Part model, mm, in its own coordinate system. Face numbers are marked on the shaded views. A direction names the side the tool comes from. Coordinates: 2 decimals unless noted, no trailing zeros. Write each loop counter-clockwise with the first axis right and the second up, starting at its lowest first coordinate (ties: lowest second). Pieces come first, ordered by that corner, then holes. Notation, with made-up numbers: (-9.75, 87) -> (49.25, 87) arc R25 cw to (49.25, 104) -> close; hole circle Ø9 at (51.5, 2). An arc over 180 degrees is marked (long way). Write item = value, one per line.
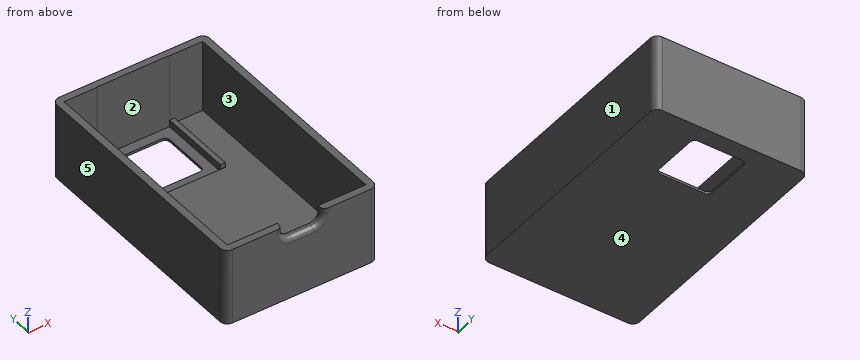
from build123d import *

# Parameters (mm, degrees)
F0_W      = 32
F0_H      = 51.5
F1_DEPTH  = 1
F2_DEPTH  = 16
F3_R      = 1.5
F4_W      = 8.5
F4_H      = 3
F5_DEPTH  = 5
F6_R      = 2
F7_R      = 1
F0_W_2    = 15.2
F0_H_2    = 13.6
F0_W_3    = 11.1999999404
F0_H_3    = 11.1999999404
F0_H_4    = 0.1
F0_H_5    = 1.5
F8_DEPTH  = 0.5
F9_R      = 1
F10_W     = 1
F10_H     = 15.1
F11_DEPTH = 1


with BuildPart() as f1:
    # F0 (on Top) → F1 (new body)
    with BuildSketch(Plane.XY):
        Rectangle(F0_W, F0_H)
        Polygon((7.6, 24.35), (7.6, 24.25), (14.5, 24.25), (14.5, -24.25), (-14.5, -24.25), (-14.5, 24.25), (-7.6, 24.25), (-7.6, 24.35), align=None, mode=Mode.SUBTRACT)
        Polygon((13, 22.75), (13, -22.75), (-13, -22.75), (-13, 22.75), (-7.6, 22.75), (-7.6, 24.25), (-14.5, 24.25), (-14.5, -24.25), (14.5, -24.25), (14.5, 24.25), (7.6, 24.25), (7.6, 22.75), align=None)
        Polygon((-13, -22.75), (13, -22.75), (13, 22.75), (7.6, 22.75), (7.6, 9.15), (-7.6, 9.15), (-7.6, 22.75), (-13, 22.75), align=None)
    extrude(amount=F1_DEPTH)

    # F0 (on Top) → F2 (join)
    with BuildSketch(Plane.XY):
        Rectangle(F0_W, F0_H)
        Polygon((7.6, 24.35), (7.6, 24.25), (14.5, 24.25), (14.5, -24.25), (-14.5, -24.25), (-14.5, 24.25), (-7.6, 24.25), (-7.6, 24.35), align=None, mode=Mode.SUBTRACT)
    extrude(amount=F2_DEPTH)

    # F3
    f3_edges = [f1.edges().sort_by_distance(p)[0] for p in [
        (-16, -25.75, 8),
        (16, -25.75, 8),
        (-16, 25.75, 8),
        (16, 25.75, 8),
    ]]
    fillet(f3_edges, radius=F3_R)

    # F4 (on face) → F5 (cut)
    with BuildSketch(Plane.XZ.offset(25.75)):
        with Locations((0.25, 14.5)):
            Rectangle(F4_W, F4_H)
    extrude(amount=-F5_DEPTH, mode=Mode.SUBTRACT)

    # F6
    f6_edges = [f1.edges().sort_by_distance(p)[0] for p in [
        (-4, -25, 13),
        (4.5, -25, 13),
    ]]
    fillet(f6_edges, radius=F6_R)

    # F7
    f7_edges = [f1.edges().sort_by_distance(p)[0] for p in [
        (-3.414214, -25.75, 13.585786),
        (0.25, -25.75, 13),
    ]]
    fillet(f7_edges, radius=F7_R)

    # F0 (on Top) → F8 (join)
    with BuildSketch(Plane.XY):
        with Locations((0, 15.95)):
            Rectangle(F0_W_2, F0_H_2)
        with Locations((0, 16.75)):
            Rectangle(F0_W_3, F0_H_3, mode=Mode.SUBTRACT)
        with Locations((0, 24.3)):
            Rectangle(F0_W_2, F0_H_4)
        with Locations((0, 23.5)):
            Rectangle(F0_W_2, F0_H_5)
    extrude(amount=F8_DEPTH)

    # F9
    f9_edges = [f1.edges().sort_by_distance(p)[0] for p in [
        (5.6, 11.15, 0.25),
        (-5.6, 11.15, 0.25),
        (5.6, 22.35, 0.25),
        (-5.6, 22.35, 0.25),
    ]]
    fillet(f9_edges, radius=F9_R)

    # F10 (on face) → F11 (join)
    with BuildSketch(Plane.XY.offset(1)):
        with Locations((-8.1, 16.7)):
            Rectangle(F10_W, F10_H)
        with Locations((8.1, 16.7)):
            Rectangle(F10_W, F10_H)
    extrude(amount=F11_DEPTH)


solid = f1.part
Q1. Saw through at A-A on z = 10. Give the cut face in (x, y), and give its area (3 significant figures).
Model answer:
outline = (-16, -24.25) arc R1.5 ccw to (-14.5, -25.75) -> (14.5, -25.75) arc R1.5 ccw to (16, -24.25) -> (16, 24.25) arc R1.5 ccw to (14.5, 25.75) -> (-14.5, 25.75) arc R1.5 ccw to (-16, 24.25) -> close; hole (-14.5, -24.25) -> (14.5, -24.25) -> (14.5, 24.25) -> (7.6, 24.25) -> (7.6, 24.35) -> (-7.6, 24.35) -> (-7.6, 24.25) -> (-14.5, 24.25) -> close
area = 238 mm²
Q2. Pin check, flat tip, straight feed: pin 1 (12 mm diameter, centred on x = -1.5, y = 10, fed in from +Z). Stop position of the tip, or through.
Model answer:
pin_1 = 1
Q3. Which spindle directions (+Z, -Z, +X, -X, +Y, -Y) get a long thin tool onto all of the face, cutting with end or side? Do the marked faces 1 and 2. Say none if no direction does.
Model answer:
face_1 = +Z, -Z, +X, +Y, -Y
face_2 = +Z
Q4. Saw through at B-B on y = -2. Give the cut face in (x, z).
Model answer:
outline = (-16, 0) -> (16, 0) -> (16, 16) -> (14.5, 16) -> (14.5, 1) -> (-14.5, 1) -> (-14.5, 16) -> (-16, 16) -> close
Q5. Saw through at C-C on x = 12.5. Give the cut face in (y, z), and give its area (3 significant figures).
Model answer:
outline = (-25.75, 0) -> (25.75, 0) -> (25.75, 16) -> (24.25, 16) -> (24.25, 1) -> (-24.25, 1) -> (-24.25, 16) -> (-25.75, 16) -> close
area = 96.5 mm²
Q6. Probe line 1 (X direction, y = -20, z = 9.5); line 2 (Y direction, x = -11.5, z = 4); line 3 (Y direction, x = 7.5, z = 9.75). List the from-to ranges inside material, lowest first. Write a range as from..to.
Model answer:
line_1 = -16..-14.5, 14.5..16
line_2 = -25.75..-24.25, 24.25..25.75
line_3 = -25.75..-24.25, 24.35..25.75
Q7. Mould opens along X. For the marked faces 3, 4 and 5 say: released by +X, released by -X, zero draft, split by the parting line, or undercut.
Model answer:
face_3 = undercut
face_4 = zero draft
face_5 = released by -X
